Geometry check sheet. Reference: the model listing, model coordinates, mm. Face numbers are marked on the shaded views. Coordinates: 2 decimals unless noted, no trailing zeros. Answer as CSV lines item,"result". Start each with the question number.
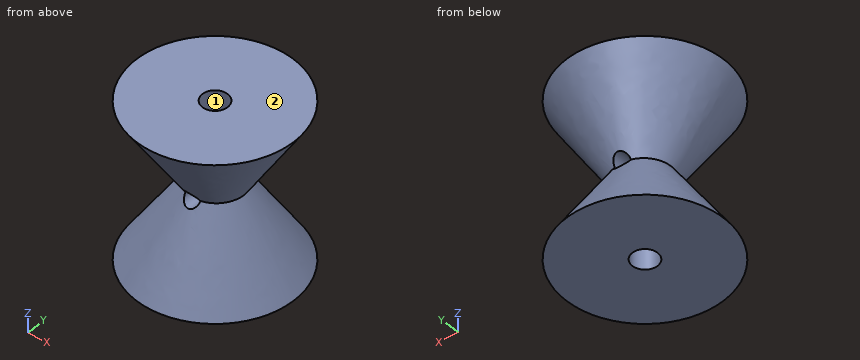
from build123d import *

# Parameters (mm, degrees)
F0_R     = 37.5
F2_R     = 13.125
F5_R     = 6
F6_DEPTH = 75.001
F7_R     = 3.75
F8_DEPTH = 37.501
F9_DEPTH = 37.501


with BuildPart() as f3:
    # F0 (on Top) → F3 section 0
    with BuildSketch(Plane.XY):
        Circle(F0_R)
    # F2 (on offset) → F3 section 1
    with BuildSketch(Plane.XY.offset(37.5)):
        with Locations((0.643553, 0)):
            Circle(F2_R)
    loft()

    # F4: F3 across plane


with BuildPart() as f3_1:
    add(f3.part)
    add(f3.part.mirror(Plane.XY.offset(37.5)))

    # F5 (on face) → F6 (cut, through all)
    with BuildSketch(Plane.XY.offset(75)):
        Circle(F5_R)
    extrude(amount=-F6_DEPTH, mode=Mode.SUBTRACT)

    # F7 (on Front) → F8 (cut, through all)
    with BuildSketch(Plane.XZ):
        with Locations((0, 37.5)):
            Circle(F7_R)
    extrude(amount=-F8_DEPTH, mode=Mode.SUBTRACT)

    # F7 (on Front) → F9 (cut, through all)
    with BuildSketch(Plane.XZ):
        with Locations((0, 37.5)):
            Circle(F7_R)
    extrude(amount=F9_DEPTH, mode=Mode.SUBTRACT)


solid = f3_1.part
Q1. Thickness scan on L1, parallel to Z at x = 0, y = -8.5; L2, parallel to Y at x = 2, z = 49; L3, parallel to X at y = 12, z = 37. Record the ranges inside material, lowest first.
Q2. Go/stop test with flat-tipped pins: pin 1 Ø1.5 at (y, z) = (0.5, 40) entering from -X; pin 2 Ø12 at (x, z) = (0, 37.5) entering from +Y; pin 3 Ø7 at (x, z) = (0, 37.5) entering from -Y; pin 4 Ø5 at (x, z) = (-1, 15.5) entering from -Y. Record where each tip stops, or that it passes through.
Q3. Release check for a two-part mould opening along Y. For the marked faces 1 and 2 record: released by +Y, released by -Y, zero draft, split by the parting line, or undercut.
Q4. Sectioned sample at A-A, the plane x = 2.5. Give the number of separate pieces and of enclosed holes in the cut face, then the cut area to 3 significant figures.
Geometry results:
1,L1,"z = 0 to 33.75, 41.25 to 75"
1,L2,"y = -20.54 to -5.66, 5.66 to 20.54"
1,L3,"x = -5.44 to -3.72, 3.72 to 6.71"
2,pin 1,"stops at x = -14.64"
2,pin 2,"stops at y = 17.02"
2,pin 3,"passes through"
2,pin 4,"stops at y = -29.03"
3,face 1,"undercut"
3,face 2,"zero draft"
4,separate pieces,"4"
4,enclosed holes,"0"
4,area,"2,870 mm^2"
